Design review of the part shown in the three views and the two pictorial views. Dimensions are in mm from the part's minimum x, y and z. Round coordinates to 2 decimals unless told otherwise and drop trailing zeros. Loops run counter-clockwise (first coordinate to the right, second up) from the corner with the lowest first, then second, coordinate; pieces in that order, holes last.
1. Consider section C-C on z = 2.1. State the section outline as (x, y) points.
2. Draft analysis for pull direction X (two halves, no side actions). For the marked faces 1, 2, 3 and 4, state which applies: released by +X, released by -X, zero draft, split by the parting line, or undercut.
3. Consider section A-A on y = 6.35. State the section outline as (x, z) points.
4. Clearance check with flat-ended pins moving along their axes: pin 1 Ø2 at (y, z) = (5, 4.5) entering from +X; pin 2 Ø1 at (y, z) = (3, 1.5) entering from +X; pin 3 Ø6 at (x, y) = (6.35, 6.35) entering from +Z. State where each tip first meets the part, or that it passes through.
5. To check wall thickness, follow line 1 along Y through (x, z) = (6.35, 4.25); line 2 along Y through (x, z) = (6.25, 1.2); line 3 along Z through (x, y) = (12, 6). State the ranges of each line that lie inside material, in increasing order.
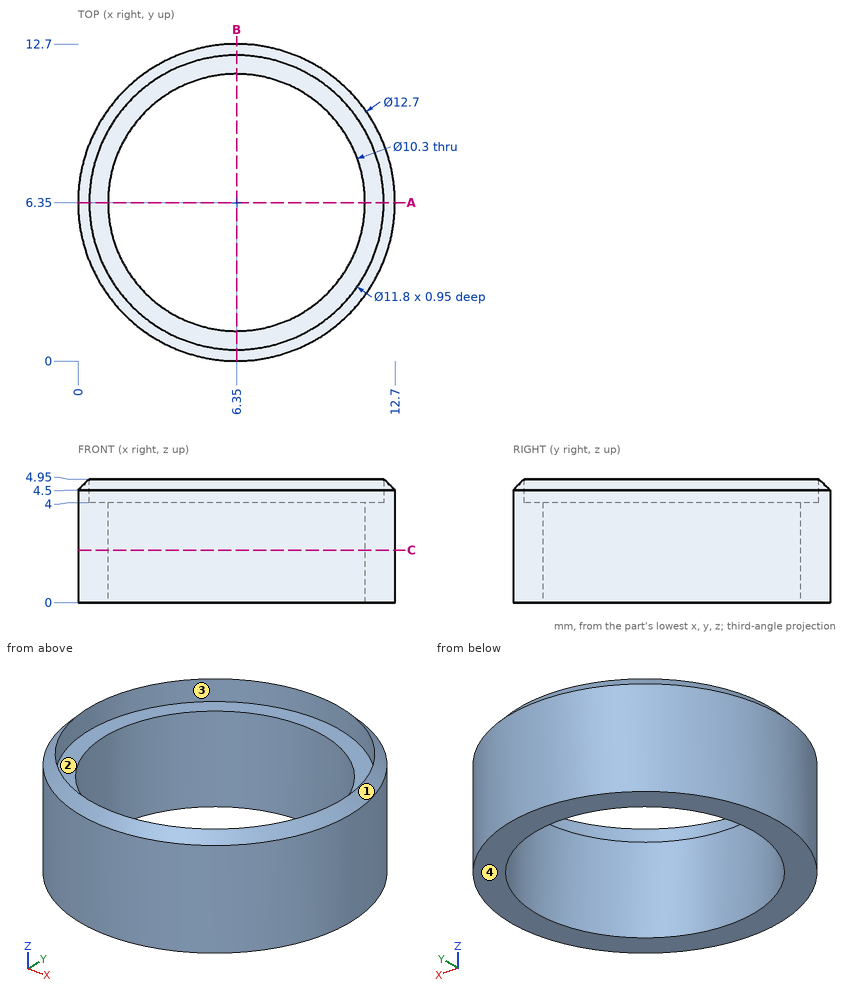
Resolved:
1. outline: circle Ø12.7 at (6.35, 6.35); hole circle Ø10.3 at (6.35, 6.35)
2. face 1: split by the parting line
2. face 2: undercut
2. face 3: undercut
2. face 4: zero draft
3. outline: (0, 0) - (1.2, 0) - (1.2, 4) - (0.45, 4) - (0.45, 4.95) - (0, 4.5) - close; (11.5, 0) - (12.7, 0) - (12.7, 4.5) - (12.25, 4.95) - (12.25, 4) - (11.5, 4) - close
4. pin 1: stops at x = 12.69
4. pin 2: stops at x = 12.02
4. pin 3: passes through
5. line 1: y = 0 to 0.45, 12.25 to 12.7
5. line 2: y = 0 to 1.2, 11.5 to 12.7
5. line 3: z = 0 to 4
